Input: dimensioned drawing with shaded views. Units: mm. Origin: part minimum x, y, z. A direction names the side the tool comes from. Give positions to 0.01 mm unless a question says otherwise; leave off trailing zeros. Order: outer loops, then holes, each group sorted by start corner. A loop starts at its lowest first (then second) coordinate and runs counter-clockwise, first axis right, second up. Notation, with made-up numbers: (-33.5, -29.75) - (-15.5, -29.75) arc R13 cw to (-15.5, -11.75) - close; hole circle Ø9 at (36.25, -38.5). An arc over 180 degrees is marked (long way). Use a Markdown table: item, result.
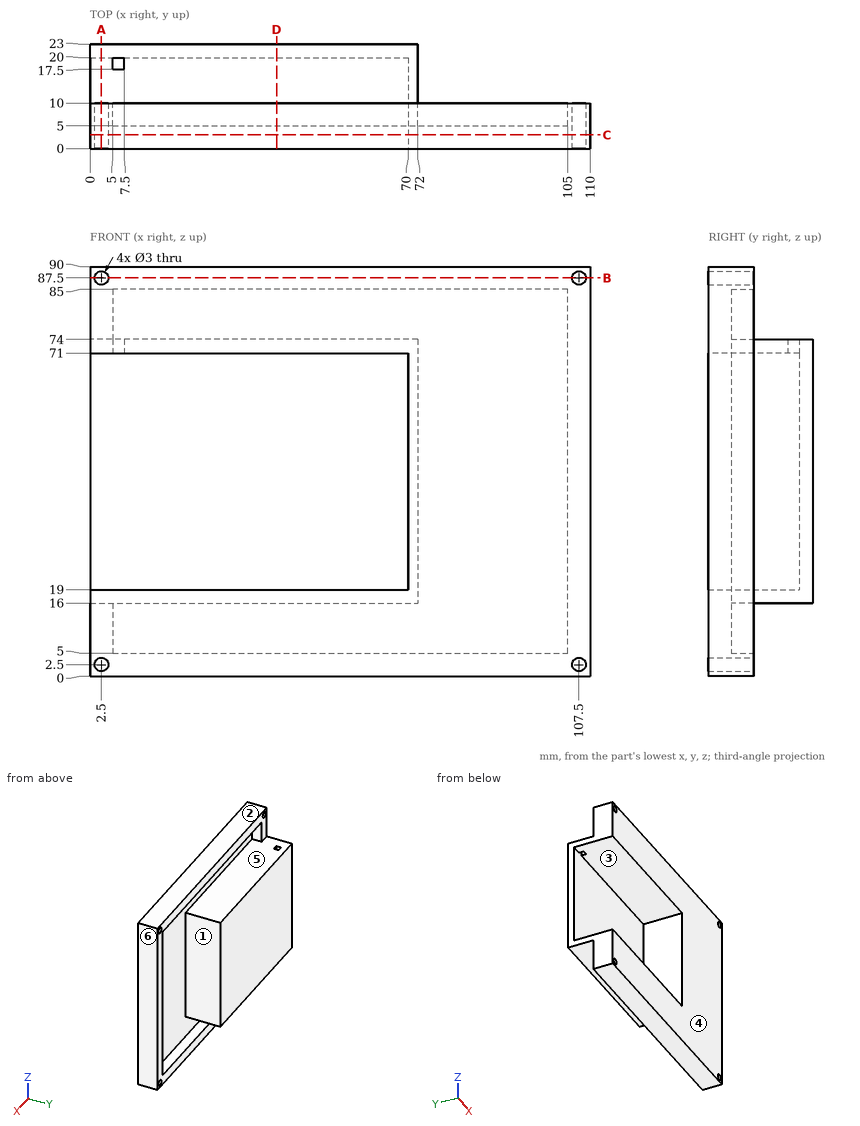
1. Section query B-B (z = 87.5). Return loops of the section in (x, y), then the cut area to 3 significant figures.
Response:
| item | result |
|---|---|
| outline | (0, 0) - (1, 0) - (1, 10) - (0, 10) - close; (4, 0) - (106, 0) - (106, 10) - (4, 10) - close; (109, 0) - (110, 0) - (110, 10) - (109, 10) - close |
| area | 1,040 mm^2 |
2. Material intervals for line 1 along Z through (x, y) = (37, 6.75); line 2 along X through (y, z) = (6.75, 87.5); line 3 along Z through (x, y) = (2.5, 2.25), sorted ascending.
Response:
| item | result |
|---|---|
| line 1 | z = 0 to 5, 16 to 19, 71 to 74, 85 to 90 |
| line 2 | x = 0 to 1, 4 to 106, 109 to 110 |
| line 3 | z = 0 to 1, 4 to 19, 71 to 86, 89 to 90 |
3. Section query C-C (y = 3). Return loops of the section in (x, z), then the cut area to 3 significant figures.
Response:
| item | result |
|---|---|
| outline | (0, 0) - (110, 0) - (110, 90) - (0, 90) - (0, 71) - (70, 71) - (70, 19) - (0, 19) - close; hole circle Ø3 at (2.5, 2.5); hole circle Ø3 at (2.5, 87.5); hole circle Ø3 at (107.5, 2.5); hole circle Ø3 at (107.5, 87.5) |
| area | 6,230 mm^2 |
4. Section query A-A (x = 2.5). Return loops of the section in (y, z), then the cut area to 3 significant figures.
Response:
| item | result |
|---|---|
| outline | (0, 0) - (10, 0) - (10, 1) - (0, 1) - close; (0, 4) - (10, 4) - (10, 16) - (23, 16) - (23, 74) - (10, 74) - (10, 86) - (0, 86) - (0, 71) - (20, 71) - (20, 19) - (0, 19) - close; (0, 89) - (10, 89) - (10, 90) - (0, 90) - close |
| area | 554 mm^2 |
5. Set-up query: the marked faces 1, 2 and 3. Return all of +Z, -Z, +X, -X, +Y, -Y with unobstructed straight access to the full face (end or side cutting, diameter ignored); none if empty.
Response:
| item | result |
|---|---|
| face 1 | +Y |
| face 2 | +Z, +X, -X, +Y, -Y |
| face 3 | -X, -Y |
6. Mould query, pull axis X, two halves, no side actions, for the marked faces 4, 5 and 6. Classes: pulls with the +X half, pulls with the -X half, needs draft (parallel to the pull), parting line crosses it, or undercut.
Response:
| item | result |
|---|---|
| face 4 | needs draft |
| face 5 | undercut |
| face 6 | pulls with the +X half |
7. Pin query (flat end, axial travel): pin 1 (16.5 mm diameter, centred on x = 40.5, z = 44, fed in from -Y); pin 2 (6 mm diameter, centred on y = 15, z = 24.5, fed in from -X); pin 3 (4 mm diameter, centred on x = 22, y = 20, fed in from -Z). Return the tip coordinate at first contact, or that it passes through.
Response:
| item | result |
|---|---|
| pin 1 | stops at y = 20 |
| pin 2 | stops at x = 70 |
| pin 3 | stops at z = 16 |
8. Section query D-D (x = 41). Return loops of the section in (y, z).
Response:
| item | result |
|---|---|
| outline | (0, 0) - (10, 0) - (10, 5) - (5, 5) - (5, 16) - (23, 16) - (23, 74) - (5, 74) - (5, 85) - (10, 85) - (10, 90) - (0, 90) - (0, 71) - (20, 71) - (20, 19) - (0, 19) - close |
